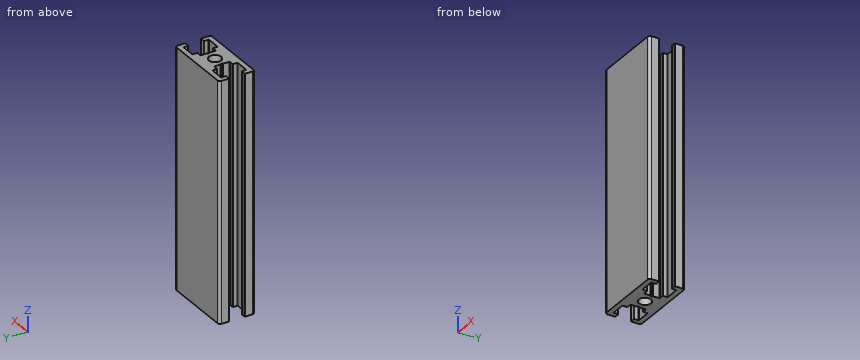
```python
from build123d import *

# Parameters (mm, degrees)
SKETCH_1_R      = 2.6
EXTRUDE_1_DEPTH = 100


with BuildPart() as part:
    # 草图1 → 凸台-拉伸1 (new body)
    with BuildSketch(Plane.XY):
        with BuildLine():
            Line((-4.7, 0.5), (-4.2, 0))
            Line((-4.2, 0), (-4.7, -0.5))
            Line((-4.7, -0.5), (-4.7, -3.05))
            ThreePointArc((-4.7, -3.05), (-4.758578644, -3.191421356), (-4.9, -3.25))
            Line((-4.9, -3.25), (-6.6, -3.25))
            ThreePointArc((-6.6, -3.25), (-6.741421356, -3.308578644), (-6.8, -3.45))
            Line((-6.8, -3.45), (-6.8, -5.1))
            ThreePointArc((-6.8, -5.1), (-6.858578644, -5.241421356), (-7, -5.3))
            Line((-7, -5.3), (-12.65, -5.3))
            ThreePointArc((-12.65, -5.3), (-12.791421356, -5.241421356), (-12.85, -5.1))
            Line((-12.85, -5.1), (-12.85, -3.45))
            ThreePointArc((-12.85, -3.45), (-12.908578644, -3.308578644), (-13.05, -3.25))
            Line((-13.05, -3.25), (-14.8, -3.25))
            ThreePointArc((-14.8, -3.25), (-14.941421356, -3.308578644), (-15, -3.45))
            Line((-15, -3.45), (-15, -6.5))
            ThreePointArc((-15, -6.5), (-14.707106781, -7.207106781), (-14, -7.5))
            Line((-14, -7.5), (14, -7.5))
            ThreePointArc((14, -7.5), (14.707106781, -7.207106781), (15, -6.5))
            Line((15, -6.5), (15, -3.45))
            ThreePointArc((15, -3.45), (14.941421356, -3.308578644), (14.8, -3.25))
            Line((14.8, -3.25), (13.05, -3.25))
            ThreePointArc((13.05, -3.25), (12.908578644, -3.308578644), (12.85, -3.45))
            Line((12.85, -3.45), (12.85, -5.1))
            ThreePointArc((12.85, -5.1), (12.791421356, -5.241421356), (12.65, -5.3))
            Line((12.65, -5.3), (7, -5.3))
            ThreePointArc((7, -5.3), (6.858578644, -5.241421356), (6.8, -5.1))
            Line((6.8, -5.1), (6.8, -3.45))
            ThreePointArc((6.8, -3.45), (6.741421356, -3.308578644), (6.6, -3.25))
            Line((6.6, -3.25), (4.9, -3.25))
            ThreePointArc((4.9, -3.25), (4.758578644, -3.191421356), (4.7, -3.05))
            Line((4.7, -3.05), (4.7, -0.5))
            Line((4.7, -0.5), (4.2, 0))
            Line((4.2, 0), (4.7, 0.5))
            Line((4.7, 0.5), (4.7, 3.05))
            ThreePointArc((4.7, 3.05), (4.758578644, 3.191421356), (4.9, 3.25))
            Line((4.9, 3.25), (6.6, 3.25))
            ThreePointArc((6.6, 3.25), (6.741421356, 3.308578644), (6.8, 3.45))
            Line((6.8, 3.45), (6.8, 5.1))
            ThreePointArc((6.8, 5.1), (6.858578644, 5.241421356), (7, 5.3))
            Line((7, 5.3), (12.65, 5.3))
            ThreePointArc((12.65, 5.3), (12.791421356, 5.241421356), (12.85, 5.1))
            Line((12.85, 5.1), (12.85, 3.45))
            ThreePointArc((12.85, 3.45), (12.908578644, 3.308578644), (13.05, 3.25))
            Line((13.05, 3.25), (14.8, 3.25))
            ThreePointArc((14.8, 3.25), (14.941421356, 3.308578644), (15, 3.45))
            Line((15, 3.45), (15, 6.5))
            ThreePointArc((15, 6.5), (14.707106781, 7.207106781), (14, 7.5))
            Line((14, 7.5), (-14, 7.5))
            ThreePointArc((-14, 7.5), (-14.707106781, 7.207106781), (-15, 6.5))
            Line((-15, 6.5), (-15, 3.45))
            ThreePointArc((-15, 3.45), (-14.941421356, 3.308578644), (-14.8, 3.25))
            Line((-14.8, 3.25), (-13.05, 3.25))
            ThreePointArc((-13.05, 3.25), (-12.908578644, 3.308578644), (-12.85, 3.45))
            Line((-12.85, 3.45), (-12.85, 5.1))
            ThreePointArc((-12.85, 5.1), (-12.791421356, 5.241421356), (-12.65, 5.3))
            Line((-12.65, 5.3), (-7, 5.3))
            ThreePointArc((-7, 5.3), (-6.858578644, 5.241421356), (-6.8, 5.1))
            Line((-6.8, 5.1), (-6.8, 3.45))
            ThreePointArc((-6.8, 3.45), (-6.741421356, 3.308578644), (-6.6, 3.25))
            Line((-6.6, 3.25), (-4.9, 3.25))
            ThreePointArc((-4.9, 3.25), (-4.758578644, 3.191421356), (-4.7, 3.05))
            Line((-4.7, 3.05), (-4.7, 0.5))
        make_face()
        Circle(SKETCH_1_R, mode=Mode.SUBTRACT)
    extrude(amount=EXTRUDE_1_DEPTH)


solid = part.part
```
The listing builds one solid part. Answer for the finished solid, in the listing's coordinates (mm). Coordinates: 2 decimals unless noted, no trailing zeros. Loops run counter-clockwise (first coordinate to the right, second up) from the corner with the lowest first, then second, coordinate; pieces in that order, holes last. Notation, with made-up numbers: M -31.75,79.25 L -1.75,79.25 A3 ccw -1.75,84.25 Z; hole C 31,-15.75 d8. An arc over 180 degrees is marked long. Answer as a JSON object with one key per item and string values. Group by question number.
Item 1: This flat-tipped pin is pushed along its axis until it touches: P1, Ø1, axis at y = 2.5, z = 19, coming from the +X side. Where does it stop, or does it pass through?
Item 2: Section B-B (x = 0) is taken. Write down the section's boundary in (y, z), and give its area (3 significant figures).
Item 3: Section A-A (x = 8) is taken. Write down the section's boundary in (y, z).
Item 4: Consider L1, parallel to X at y = 5, z = 43.5; L2, parallel to Y at x = 0, z = 25; L3, parallel to Y at x = -8, z = 76.5. Determine where each line is inside the solid, lowest interval first.
Solved:
{
 "1": {"P1": "stops at x = 4.7"},
 "2": {"outline": "M -7.5,0 L -2.6,0 L -2.6,100 L -7.5,100 Z; M 2.6,0 L 7.5,0 L 7.5,100 L 2.6,100 Z", "area": "980 mm2"},
 "3": {"outline": "M -7.5,0 L -5.3,0 L -5.3,100 L -7.5,100 Z; M 5.3,0 L 7.5,0 L 7.5,100 L 5.3,100 Z"},
 "4": {"L1": "x = -15 to -12.85, -6.8 to 6.8, 12.85 to 15", "L2": "y = -7.5 to -2.6, 2.6 to 7.5", "L3": "y = -7.5 to -5.3, 5.3 to 7.5"}
}
